The model under review builds one solid part; all positions refer to its coordinate system, in mm. A direction names the side the tool comes from. Give positions to 0.01 mm unless a question says otherwise; leave off trailing zeros. Write each loop counter-clockwise with the first axis right and the second up, starting at its lowest first coordinate (ties: lowest second). Pieces come first, ordered by that corner, then holes.
Autodesk Inventor part; units mm, degrees
ref_plane "YZ Plane" through (0, 0, 0) normal (1, 0, 0) x (0, 1, 0)
ref_plane "XZ Plane" through (0, 0, 0) normal (0, 1, 0) x (-1, 0, 0)
ref_plane "XY Plane" through (0, 0, 0) normal (0, 0, 1) x (1, 0, 0)
sketch "Sketch1" plane through (0, 0, 0) normal (0, 0, 1) x (1, 0, 0)
  line L0 (0, 38.5) -> (0, -38.5) construction
  line L1 (-38.5, 0) -> (38.5, 0) construction
  line L2 (-27.5, 27.5) -> (27.5, 27.5)
  line L3 (27.5, 27.5) -> (27.5, -27.5)
  line L4 (27.5, -27.5) -> (-27.5, -27.5)
  line L5 (-27.5, -27.5) -> (-27.5, 27.5)
  point P0 (0, 0)
  dimension "d0" = 55
  dimension "d1" = 55
extrude "Extrusion1" add sketch "Sketch1" along normal blind 20
sketch "Sketch4" plane through (0, 0, 20) normal (0, 0, 1) x (1, 0, 0)
  line L0 (-38.5, 0) -> (38.5, 0) construction
  line L1 (0, 38.5) -> (0, -38.5) construction
  line L2 (-22.55, 22.55) -> (22.55, 22.55) construction
  line L3 (22.55, 22.55) -> (22.55, -22.55) construction
  line L4 (22.55, -22.55) -> (-22.55, -22.55) construction
  line L5 (-22.55, -22.55) -> (-22.55, 22.55) construction
  point P0 (0, 0)
  dimension "d15" = 45.1
  dimension "d16" = 45.1
hole "Hole2" at (-22.55, 22.55, 20) at (22.55, 22.55, 20) at (22.55, -22.55, 20) at (-22.55, -22.55, 20) at (-22.55, 22.55, 20) at (22.55, 22.55, 20) direction (0, 0, -1) diameter 5 depth 8
sketch "Sketch5" plane through (0, 0, 20) normal (0, 0, 1) x (1, 0, 0)
  circle A0 centre (-22.55, 22.55) radius 2.5
  circle A1 centre (22.55, -22.55) radius 2.5
  line L0 (-22.55, 22.55) -> (22.55, 22.55)
  line L1 (22.55, 22.55) -> (22.55, -22.55)
  line L2 (22.55, -22.55) -> (-22.55, -22.55)
  line L3 (-22.55, -22.55) -> (-22.55, 22.55)
  point P0 (0, 0)
extrude "Extrusion3" cut sketch "Sketch5" against normal blind 8 contours L0 L1 A1 L2 L3 A0 | A0 L3 L0 | L1 L2 A1 picked at (-20.9042, 22.3646) picked at (22.003, -20.9868)
sketch "Sketch6" plane through (-27.5, -27.5, 0) normal (-1, 0, 0) x (0, 0, 1)
  line L0 (0, 55) -> (20, 55)
  line L1 (0, 0) -> (20, 0)
  line L2 (20, 7.45) -> (12, 7.45) construction
  line L3 (20, 47.55) -> (20, 7.45) construction
  line L4 (12, 47.55) -> (20, 47.55) construction
  line L5 (12, 7.45) -> (12, 47.55) construction
  line L6 (16, 47.55) -> (16, 7.45) construction
  point P0 (0, 27.5)
  point P1 (16, 40)
  point P2 (16, 15)
  dimension "d26" = 15
  dimension "d27" = 15
hole "Hole3" at (-27.5, 12.5, 16) at (-27.5, -12.5, 16) direction (1, 0, 0) diameter 3.242 end up to surface
sketch "Sketch8" plane through (0, 0, 0) normal (0, 0, -1) x (-1, 0, 0)
  line L0 (27.5, 27.5) -> (-27.5, 27.5) construction
  line L1 (-27.5, 27.5) -> (-27.5, -27.5) construction
  line L2 (-27.5, -27.5) -> (27.5, -27.5) construction
  line L3 (27.5, -27.5) -> (27.5, 27.5) construction
  line L4 (0, -38.5) -> (0, 38.5) construction
  line L5 (-38.5, 0) -> (38.5, 0) construction
  line L6 (-12.5, -12.5) -> (12.5, -12.5)
  line L7 (12.5, -12.5) -> (12.5, 12.5)
  line L8 (12.5, 12.5) -> (-12.5, 12.5)
  line L9 (-12.5, 12.5) -> (-12.5, -12.5)
  point P0 (0, 0)
  dimension "d44" = 25
  dimension "d45" = 25
extrude "Extrusion4" cut sketch "Sketch8" against normal blind 6
sketch "Sketch9" plane through (0, 0, 0) normal (0, 0, -1) x (-1, 0, 0)
  line L0 (12.5, 12.5) -> (12.5, -12.5) construction
  line L1 (12.5, -12.5) -> (-12.5, -12.5) construction
  line L2 (-12.5, -12.5) -> (-12.5, 12.5) construction
  line L3 (-12.5, 12.5) -> (12.5, 12.5) construction
  line L4 (27.5, 27.5) -> (-27.5, 27.5) construction
  line L5 (-27.5, 27.5) -> (-27.5, -27.5) construction
  line L6 (-27.5, -27.5) -> (27.5, -27.5) construction
  line L7 (27.5, -27.5) -> (27.5, 27.5) construction
  line L8 (12.5, -12.5) -> (-12.5, -12.5) construction
  point P0 (0, 0)
hole "Hole5" at (-12.5, 12.5, 0) at (-12.5, -12.5, 0) at (12.5, -12.5, 0) at (12.5, 12.5, 0) direction (0, 0, 1) diameter 3 depth 6
sketch "Sketch10" plane through (0, 0, 6) normal (0, 0, -1) x (-1, 0, 0)
  point P0 (0, 0)
  point P1 (0, 0)
hole "Hole6" at (0, 0, 6) direction (0, 0, 1) diameter 3.242 depth 4 tip angle 118
properties part number "Large-cuvette-mount-40mm-V3" material "PC/ABS Plastic"
1) Consider section D-D, the plane y = -24. Give the boundary of the cut face in (x, z), then the cut area to 3 significant figures.
2) Consider section C-C, the plane x = -17.5. Give the boundary of the cut face in (y, z).
3) Consider section A-A, the plane z = 5.25. Give the boundary of the cut face in (x, y).
4) The part is to be moulded in two halves that separate along X. For faces 1 (the flat face through (27.5, 0, 10)), 2 (the cylindrical face through (-13.595, -13.525, 3.042)), 3 (the cylindrical face through (-24.99, -12.987, 17.546)), say which applies: +X half, -X half, draft (parallel to the pull), parting line (faces both ways), or undercut.
5) Insertion check: pin 1 (4 mm diameter, centred on x = -22.55, y = 22.55, fed in from +Z); pin 2 (8.5 mm diameter, centred on x = -6.5, y = 7, fed in from -Z). Each pin has a flat end and moves straight along its axis. Give the tip position at first contact, or say it passes through.
6) Tool access review of faces 4 (the cylindrical face through (-24.375, 24.259, 15.944)), 5 (the cylindrical face through (1.438, 0.748, 8.028)), 6 (the flat face through (0, -27.5, 10)): name each direction out of +Z, -Z, +X, -X, +Y, -Y from which nothing blocks a thin tool from reaching the whole face with its end or side.
7) Consider section B-B, the plane z = 16. Give the boundary of the cut face in (x, y).
8) To check wall thickness, follow probe 1 along X at (y, z) = (2, 12.5); probe 2 along X at (y, z) = (0, 2.5); probe 3 along X at (y, z) = (-23, 18.5). State the ranges of each line that lie inside material, in increasing order.
Answer block:
1. outline: (-27.5, 0) - (27.5, 0) - (27.5, 20) - (24.59, 20) - (24.59, 12) - (20.51, 12) - (20.51, 20) - (-20.51, 20) - (-20.51, 12) - (-24.59, 12) - (-24.59, 20) - (-27.5, 20) - close
1. area: 1,030 mm2
2. outline: (-27.5, 0) - (27.5, 0) - (27.5, 20) - (22.55, 20) - (22.55, 12) - (-22.55, 12) - (-22.55, 20) - (-27.5, 20) - close
3. outline: (-27.5, -27.5) - (27.5, -27.5) - (27.5, 27.5) - (-27.5, 27.5) - close; hole (-12.5, -11) arc R1.5 ccw (long way) to (-11, -12.5) - (11, -12.5) arc R1.5 ccw (long way) to (12.5, -11) - (12.5, 11) arc R1.5 ccw (long way) to (11, 12.5) - (-11, 12.5) arc R1.5 ccw (long way) to (-12.5, 11) - close
4. face 1: +X half
4. face 2: undercut
4. face 3: draft
5. pin 1: stops at z = 12
5. pin 2: stops at z = 6
6. face 4: +Z
6. face 5: -Z
6. face 6: +Z, -Z, +X, -X, -Y
7. outline: (-27.5, -27.5) - (27.5, -27.5) - (27.5, 27.5) - (-27.5, 27.5) - (-27.5, 14.12) - (-22.55, 14.12) - (-22.55, 20.05) arc R2.5 cw (long way) to (-20.05, 22.55) - (20.05, 22.55) arc R2.5 cw (long way) to (22.55, 20.05) - (22.55, -20.05) arc R2.5 cw (long way) to (20.05, -22.55) - (-20.05, -22.55) arc R2.5 cw (long way) to (-22.55, -20.05) - (-22.55, -14.12) - (-27.5, -14.12) - close; (-27.5, -10.88) - (-22.55, -10.88) - (-22.55, 10.88) - (-27.5, 10.88) - close
8. probe 1: x = -27.5 to -22.55, 22.55 to 27.5
8. probe 2: x = -27.5 to -12.5, 12.5 to 27.5
8. probe 3: x = -27.5 to -25.01, -20.09 to 20.09, 25.01 to 27.5
